Part model, mm, in its own coordinate system. A direction names the side the tool comes from. Round coordinates to 2 decimals unless told otherwise and drop trailing zeros. Order: outer loops, then holes, each group sorted by start corner. A loop starts at its lowest first (then second) coordinate and runs counter-clockwise, first axis right, second up. Notation, with made-up numbers: (50, 7.5) - (65, 7.5) arc R5 ccw to (65, 12.5) - close; hole circle Ø10 at (13, 29). An arc over 180 degrees is marked (long way). Return JSON: item names as keys, results as strings. Group by question number.
Item 1: Probe probe 1 along Y at (x, z) = (228.25, 1360); probe 2 along X at (y, z) = (133, 475.5); probe 3 along Y at (x, z) = (45.5, 653.5). List the from-to ranges inside material, lowest first.
Item 2: Drop flat-ended pins along their axis: pin 1 (2 mm diameter, centred on x = 177.5, z = 1165, fed in from +Y); pin 2 (3 mm diameter, centred on y = 2, z = 1112, fed in from +X); pin 3 (2 mm diameter, centred on y = 2.5, z = 1274, fed in from -X); pin 4 (11 mm diameter, centred on y = 34, z = 1360, fed in from -X). Give the stop position or say it passes through.
Item 3: Tool access for faces 4 (the face through (230, 81, 683)), 5 (the face through (23, 161, 684)): list every direction of +Z, -Z, +X, -X, +Y, -Y with a clear straight run to the whole face (end or side of a thin tool).
Item 4: Saw through at A-A on y = 56. List the corners of the cut face in (x, z).
Item 5: Saw through at B-B on z = 798. List the corners of the cut face in (x, y), and give its area (3 significant figures).
Item 6: Two-plate mould, pull along X, no slides. Class faces 1 (the face through (0, 84, 683)), 2 (the face through (23, 165, 684)), 3 (the face through (4, 81, 683)): released by +X, released by -X, zero draft, split by the parting line, or undercut.
```python
from build123d import *

# Parameters (mm, degrees)
BASE_FLANGE1_DEPTH = 1385
SKETCH6_W          = 60
SKETCH6_H          = 6
CUT_EXTRUDE1_DEPTH = 1414.63007891
SKETCH7_R          = 6
CUT_EXTRUDE2_DEPTH = 1414.63007891
FILLET1_R          = 10
SKETCH8_R          = 9
SKETCH8_W          = 52.5
SKETCH8_H          = 75
CUT_EXTRUDE3_DEPTH = 10


# Sheet-metal steps are written as plain solids
with BuildPart() as part:
    # Sketch1 → Base-Flange1 (new body)
    with BuildSketch(Plane.XY):
        with BuildLine():
            Line((40, 165), (6, 165))
            ThreePointArc((6, 165), (1.757359313, 163.242640687), (0, 159))
            Line((0, 159), (0, 6))
            ThreePointArc((0, 6), (1.757359313, 1.757359313), (6, 0))
            Line((6, 0), (224, 0))
            ThreePointArc((224, 0), (228.242640687, 1.757359313), (230, 6))
            Line((230, 6), (230, 159))
            ThreePointArc((230, 159), (228.242640687, 163.242640687), (224, 165))
            Line((224, 165), (190, 165))
            Line((190, 165), (190, 161))
            Line((190, 161), (224, 161))
            ThreePointArc((224, 161), (225.414213562, 160.414213562), (226, 159))
            Line((226, 159), (226, 6))
            ThreePointArc((226, 6), (225.414213562, 4.585786438), (224, 4))
            Line((224, 4), (6, 4))
            ThreePointArc((6, 4), (4.585786438, 4.585786438), (4, 6))
            Line((4, 6), (4, 159))
            ThreePointArc((4, 159), (4.585786438, 160.414213562), (6, 161))
            Line((6, 161), (40, 161))
            Line((40, 161), (40, 165))
        make_face()
    extrude(amount=BASE_FLANGE1_DEPTH)

    # Sketch6 → Cut-Extrude1 (cut, through all)
    with BuildSketch(Plane(origin=(0, 0, 0), x_dir=(0, 0, -1), z_dir=(1, 0, 0))):
        with Locations((-30, 162)):
            Rectangle(SKETCH6_W, SKETCH6_H)
        with Locations((-1355, 162)):
            Rectangle(SKETCH6_W, SKETCH6_H)
        with Locations((-1355, 3)):
            Rectangle(SKETCH6_W, SKETCH6_H)
        with Locations((-30, 3)):
            Rectangle(SKETCH6_W, SKETCH6_H)
    extrude(amount=CUT_EXTRUDE1_DEPTH, mode=Mode.SUBTRACT)

    # Sketch7 → Cut-Extrude2 (cut, through all)
    with BuildSketch(Plane.ZY):
        with Locations(Location((25, 134, 0), (0, 0, 270))):
            Circle(SKETCH7_R)
        with Locations(Location((25, 84, 0), (0, 0, 270))):
            Circle(SKETCH7_R)
        with Locations(Location((25, 34, 0), (0, 0, 270))):
            Circle(SKETCH7_R)
        with Locations((1360, 34)):
            Circle(SKETCH7_R)
        with Locations((1360, 84)):
            Circle(SKETCH7_R)
        with Locations((1360, 134)):
            Circle(SKETCH7_R)
    extrude(amount=-CUT_EXTRUDE2_DEPTH, mode=Mode.SUBTRACT)

    # Fillet1
    fillet1_edges = [part.edges().sort_by_distance(p)[0] for p in [
        (190, 163, 1325),
        (40, 163, 1325),
        (190, 163, 60),
        (40, 163, 60),
        (228, 159, 0),
        (228, 159, 1385),
        (228, 6, 0),
        (228, 6, 1385),
        (2, 6, 0),
        (2, 6, 1385),
        (2, 159, 0),
        (2, 159, 1385),
    ]]
    fillet(fillet1_edges, radius=FILLET1_R)

    # Sketch8 → Cut-Extrude3 (cut)
    with BuildSketch(Plane(origin=(0, 4, 0), x_dir=(1, 0, 0), z_dir=(0, 1, 0))):
        with Locations(Location((85, -767.5, 0), (0, 0, 270))):
            Circle(SKETCH8_R)
        with Locations(Location((145, -737.5, 0), (0, 0, 270))):
            Circle(SKETCH8_R)
        with Locations(Location((145, -677.5, 0), (0, 0, 270))):
            Circle(SKETCH8_R)
        with Locations(Location((145, -617.5, 0), (0, 0, 270))):
            Circle(SKETCH8_R)
        with Locations(Location((85, -707.5, 0), (0, 0, 270))):
            Circle(SKETCH8_R)
        with Locations(Location((85, -647.5, 0), (0, 0, 270))):
            Circle(SKETCH8_R)
        with Locations((151.25, -1112.5)):
            Rectangle(SKETCH8_W, SKETCH8_H)
        with Locations((78.75, -1112.5)):
            Rectangle(SKETCH8_W, SKETCH8_H)
        with Locations((78.75, -272.5)):
            Rectangle(SKETCH8_W, SKETCH8_H)
        with Locations((151.25, -272.5)):
            Rectangle(SKETCH8_W, SKETCH8_H)
        with BuildLine():
            Line((190.5, -1298), (190.5, -1258))
            ThreePointArc((190.5, -1258), (197.5, -1251), (204.5, -1258))
            Line((204.5, -1258), (204.5, -1298))
            ThreePointArc((204.5, -1298), (197.5, -1305), (190.5, -1298))
        make_face()
        with BuildLine():
            Line((39.5, -1298), (39.5, -1258))
            ThreePointArc((39.5, -1258), (32.5, -1251), (25.5, -1258))
            Line((25.5, -1258), (25.5, -1298))
            ThreePointArc((25.5, -1298), (32.5, -1305), (39.5, -1298))
        make_face()
        with BuildLine():
            Line((39.5, -87), (39.5, -127))
            ThreePointArc((39.5, -127), (32.5, -134), (25.5, -127))
            Line((25.5, -127), (25.5, -87))
            ThreePointArc((25.5, -87), (32.5, -80), (39.5, -87))
        make_face()
        with BuildLine():
            Line((190.5, -87), (190.5, -127))
            ThreePointArc((190.5, -127), (197.5, -134), (204.5, -127))
            Line((204.5, -127), (204.5, -87))
            ThreePointArc((204.5, -87), (197.5, -80), (190.5, -87))
        make_face()
    extrude(amount=-CUT_EXTRUDE3_DEPTH, mode=Mode.SUBTRACT)


solid = part.part
```
Filled in:
{
 "1": {"probe 1": "y = 6 to 28, 40 to 78, 90 to 128, 140 to 159", "probe 2": "x = 0 to 4, 226 to 230", "probe 3": "y = 0 to 4"},
 "2": {"pin 1": "stops at y = 4", "pin 2": "stops at x = 229.45", "pin 3": "stops at x = 0.55", "pin 4": "passes through"},
 "3": {"face 4": "+Z, -Z, +X, +Y, -Y", "face 5": "+Z, -Z"},
 "4": {"outline": "(0, 0) - (4, 0) - (4, 1385) - (0, 1385) - close; (226, 0) - (230, 0) - (230, 1385) - (226, 1385) - close"},
 "5": {"outline": "(0, 6) arc R6 ccw to (6, 0) - (224, 0) arc R6 ccw to (230, 6) - (230, 159) arc R6 ccw to (224, 165) - (190, 165) - (190, 161) - (224, 161) arc R2 cw to (226, 159) - (226, 6) arc R2 cw to (224, 4) - (6, 4) arc R2 cw to (4, 6) - (4, 159) arc R2 cw to (6, 161) - (40, 161) - (40, 165) - (6, 165) arc R6 ccw to (0, 159) - close", "area": "2,470 mm^2"},
 "6": {"face 1": "released by -X", "face 2": "zero draft", "face 3": "undercut"}
}
